Work out the finished part from the listing and answer in its coordinate system (mm). Face numbers are marked on the shaded views. A direction names the side the tool comes from. Coordinates: 2 decimals unless noted, no trailing zeros. Order: outer loops, then holes, each group sorted by start corner. A loop starts at its lowest first (then second) coordinate and runs counter-clockwise, first axis right, second up. Notation, with made-up numbers: M 20.25,-27 L 50.25,-27 A23 ccw 50.25,9 Z; hole C 17,-7.75 d8. An arc over 180 degrees is marked long. Use a Markdown table: item, result.
from build123d import *

# Parameters (mm, degrees)
F0_R     = 52.0623730702
F1_DEPTH = 127
F1_TAPER = -20
F2_R     = 25.4
F3_SIZE  = 63.5
F4_T     = -2.54


# Not quite as in the source:
# - a shell that OpenCascade refuses in one call is made with other operations: the cavity is built on its own and cut out


with BuildPart() as f1:
    # F0 (on Front) → F1 (new body, symmetric)
    with BuildSketch(Plane.XZ):
        Circle(F0_R)
    extrude(amount=F1_DEPTH, both=True, taper=F1_TAPER)

    # F2
    f2_edges = [f1.edges().sort_by_distance(p)[0] for p in [
        (-98.286593, -127, 0),
    ]]
    fillet(f2_edges, radius=F2_R)

    # F3
    f3_edges = [f1.edges().sort_by_distance(p)[0] for p in [
        (-98.286593, 127, 0),
    ]]
    chamfer(f3_edges, length=F3_SIZE)

    # F4: a shell. OpenCascade refuses it in one call, so the cavity is built on its own and cut out:
    # the body offset inwards by the wall thickness, plus a prism from it out through each open face.
    f4_core = offset(f1.part, amount=F4_T, kind=Kind.INTERSECTION, mode=Mode.PRIVATE)
    f4_exits = [f4_core.faces().sort_by_distance(p)[0] for p in [
        (0, -124.46, 0),
    ]]
    add(f4_core, mode=Mode.SUBTRACT)
    extrude(f4_exits, amount=-F4_T, mode=Mode.SUBTRACT)


solid = f1.part
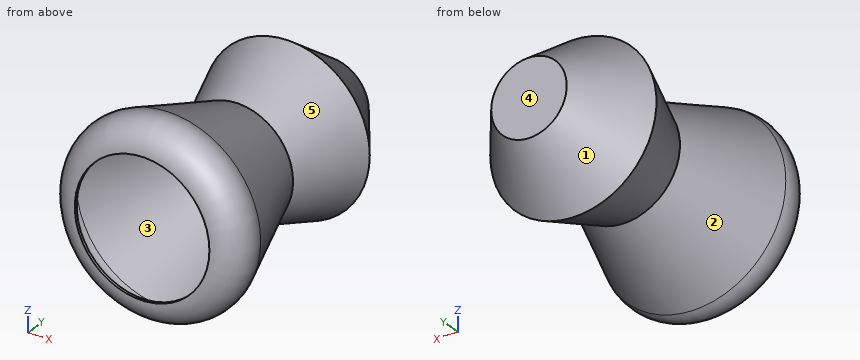
1. Find the intervals of material crossed by probe 1 along Z at (x, y) = (58, 78); probe 2 along X at (y, z) = (9, -1.5); probe 3 along Z at (x, y) = (-49, 27), in increasing order.
Answers below:
| item | result |
|---|---|
| probe 1 | -37.55 to -31.49, 31.49 to 37.55 |
| probe 2 | -55.32 to -52.61, 52.61 to 55.32 |
| probe 3 | -37.81 to -33.2, 33.2 to 37.81 |
2. For the marked faces 4 and 5, determine the directions among +Z, -Z, +X, -X, +Y, -Y from which every point of the face is accessible in a straight line to the end or side of a thin tool.
Answers below:
| item | result |
|---|---|
| face 4 | +Z, -Z, +X, -X, +Y |
| face 5 | none |
3. Section B-B on x = 0 is taken. Determine the outline of the cut face in (y, z), then the cut area to 3 significant figures.
Answers below:
| item | result |
|---|---|
| outline | M -127,-62.01 A25.4 ccw -92.91,-85.88 L 0,-52.06 L 67.33,-76.57 L 127,-34.79 L 127,34.79 L 67.33,76.57 L 0,52.06 L -92.91,85.88 A25.4 ccw -127,62.01 L -124.46,62.01 A22.86 cw -93.78,83.49 L 0,49.36 L 66.96,73.73 L 124.46,33.46 L 124.46,-33.46 L 66.96,-73.73 L 0,-49.36 L -93.78,-83.49 A22.86 cw -124.46,-62.01 Z |
| area | 1,640 mm² |
4. Section C-C on y = -36 is taken. Determine the outline of the cut face in (x, z).
Answers below:
| item | result |
|---|---|
| outline | C 0,0 d130.33; hole C 0,0 d124.92 |
5. For a pull along Y with two mould halves and no side action, classify the marked faces 1, 2 and 3 as +Y half, -Y half, draft (parallel to the pull), parting line (faces both ways), or undercut.
Answers below:
| item | result |
|---|---|
| face 1 | +Y half |
| face 2 | undercut |
| face 3 | undercut |
6. Section A-A on z = -69.5 is taken. Give the number of separate pieces and of enclosed holes in the cut face, then the cut area to 3 significant figures.
Answers below:
| item | result |
|---|---|
| separate pieces | 2 |
| enclosed holes | 2 |
| area | 1,860 mm² |
7. Flat-ended cylindrical pins translate along their axes: P1, Ø8, axis at x = 27, y = 42.5, coming from the +Z side; P2, Ø5, axis at x = -15, z = -61.5, coming from the +Y side; P3, Ø4, axis at y = 73, z = 9, coming from the -X side. Find the tip coordinate at first contact, or state that the pin passes through.
Answers below:
| item | result |
|---|---|
| P1 | z = 64.16 |
| P2 | y = 89.84 |
| P3 | x = -73.47 |
